The model under review builds one solid part; all positions refer to its coordinate system, in mm. Give positions to 0.01 mm unless a question says otherwise; leave off trailing zeros. Order: outer loops, then holes, each group sorted by start corner. A loop starts at its lowest first (then second) coordinate and runs counter-clockwise, first axis right, second up.
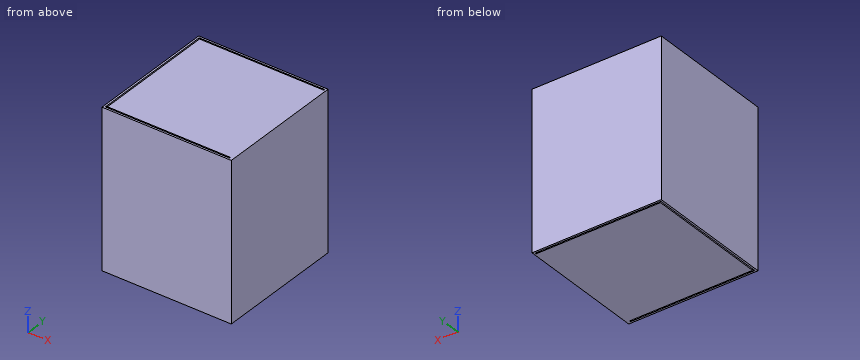
Autodesk Inventor part; units mm, degrees
ref_plane "YZ Plane" through (0, 0, 0) normal (1, 0, 0) x (0, 1, 0)
ref_plane "XZ Plane" through (0, 0, 0) normal (0, 1, 0) x (-1, 0, 0)
ref_plane "XY Plane" through (0, 0, 0) normal (0, 0, 1) x (1, 0, 0)
sketch "Boceto1" plane through (0, 0, 0) normal (0, 0, 1) x (1, 0, 0)
  line L0 (-200, -197.9) -> (-200, 0)
  line L1 (-198, 0) -> (-198, -197.9)
  line L2 (-200, 0) -> (-198, 0)
  line L3 (-197.9, 0) -> (0, 0)
  line L4 (0, -2) -> (-197.9, -2)
  line L5 (0, 0) -> (0, -2)
  line L6 (0, -2.1) -> (0, -200)
  line L7 (-2, -200) -> (-2, -2.1)
  line L8 (0, -200) -> (-2, -200)
  line L9 (-2.1, -200) -> (-200, -200)
  line L10 (-200, -198) -> (-2.1, -198)
  line L11 (-200, -200) -> (-200, -198)
  line L12 (-200, -200) -> (0, -200)
  line L13 (0, -200) -> (0, 0)
  line L14 (0, 0) -> (-200, 0)
  line L15 (-200, 0) -> (-200, -200)
  line L16 (0, 0) -> (0, 3)
  line L17 (0, 3) -> (3, 3)
  line L18 (-200, -200) -> (-203, -200)
  line L19 (-203, -200) -> (-203, -203)
  line L20 (-203, -203) -> (3, -203)
  line L21 (3, -203) -> (3, 3)
  line L22 (3, 3) -> (-203, 3)
  line L23 (-203, 3) -> (-203, -203)
  line L24 (-200, -197.9) -> (-198, -197.9)
  line L25 (-197.9, 0) -> (-197.9, -2)
  line L26 (0, -2.1) -> (-2, -2.1)
  line L27 (-2.1, -200) -> (-2.1, -198)
  point P0 (-198, -198)
  point P1 (-198, -2)
  point P2 (-2, -2)
  point P3 (-2, -198)
  dimension "espesor" = 3
  dimension "d1" = 3
  dimension "d2" = 3
  dimension "d3" = 3
extrude "Extrusión1" add sketch "Boceto1" along normal blind 220 and the other way blind 30 contours L15 L11 L18 L23 L22 L16 L3 L14 L2 L0 | L24 L1 L14 L25 L4 L13 L26 L7 L12 L27 L10 L15 | L9 L12 L8 L6 L13 L5 L16 L17 L21 L20 L19 L18 | L7 L26 L6 L8
equation "\"d1\" = espesor"
equation "\"d2\" = espesor"
equation "\"d3\" = espesor"
properties part number "Envolvente"
Item 1: Take a section at B-B (z = 140.5). Give the boundary of the cut face in (x, y), and give its area (3 significant figures).
Values found:
outline: (-203, -203) - (3, -203) - (3, 3) - (-203, 3) - close; hole (-200, -200) - (-2.1, -200) - (-2.1, -198) - (-200, -198) - close; hole (-200, -197.9) - (-198, -197.9) - (-198, 0) - (-200, 0) - close; hole (-197.9, -2) - (0, -2) - (0, 0) - (-197.9, 0) - close
area: 41,200 mm2
Item 2: For line 1 (Y direction, x = -117.5, z = 79.5); line 2 (X direction, y = -140, z = 194), list the stretches that pass through material, from the lowest coordinate up.
Values found:
line 1: y = -203 to -200, -198 to -2, 0 to 3
line 2: x = -203 to -200, -198 to 3
Item 3: Take a section at A-A (x = -55.5). Give the boundary of the cut face in (y, z).
Values found:
outline: (-203, -30) - (-200, -30) - (-200, 220) - (-203, 220) - close; (-198, -30) - (-2, -30) - (-2, 220) - (-198, 220) - close; (0, -30) - (3, -30) - (3, 220) - (0, 220) - close
